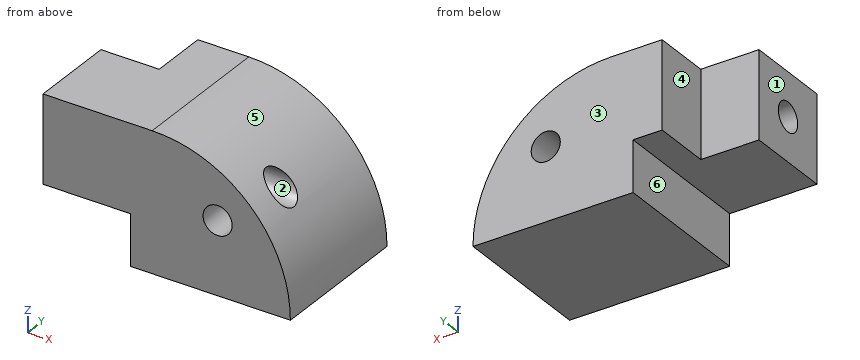
from build123d import *

# Parameters (mm, degrees)
F0_W     = 127
F0_H     = 120.65
F1_DEPTH = 215.9
F2_W     = 76.2
F2_H     = 44.45
F3_DEPTH = 127
F4_W     = 50.8
F4_H     = 76.2
F5_DEPTH = 50.8
F8_D     = 25.4
F8_DEPTH = 127
F8_TIP   = 7.6309298617
F9_R     = 120.64999
F10_D    = 25.4


# Not quite as in the source:
# - a fillet or chamfer is up to 0.001 mm smaller than in the source, because OpenCascade refuses the exact size


with BuildPart() as f1:
    # F0 (on Right) → F1 (new body)
    with BuildSketch(Plane.YZ):
        Rectangle(F0_W, F0_H)
    extrude(amount=F1_DEPTH)

    # F2 (on face) → F3 (cut)
    with BuildSketch(Plane.XZ.offset(63.5)):
        with Locations((38.1, -38.1)):
            Rectangle(F2_W, F2_H)
    extrude(amount=-F3_DEPTH, mode=Mode.SUBTRACT)

    # F4 (on face) → F5 (cut)
    with BuildSketch(Plane(origin=(0, 0, 0), x_dir=(0, -1, 0), z_dir=(-1, 0, 0))):
        with Locations((-38.1, 22.225)):
            Rectangle(F4_W, F4_H)
    extrude(amount=-F5_DEPTH, mode=Mode.SUBTRACT)

    # F8
    with Locations(Plane.XZ.offset(63.5)):
        with Locations((152.4, 3.175)):
            Hole(F8_D / 2, depth=F8_DEPTH)
            with Locations((0, 0, -(F8_DEPTH + F8_TIP / 2))):  # 118° drill point
                Cone(0, F8_D / 2, F8_TIP, mode=Mode.SUBTRACT)

    # F9 (radius 120.65 in the source; OpenCascade refuses exactly that, so slightly less here)
    f9_edges = [f1.edges().sort_by_distance(p)[0] for p in [
        (215.9, 0, 60.325),
    ]]
    fillet(f9_edges, radius=F9_R)

    # F10 (through all)
    with Locations(Plane(origin=(0, 0, 0), x_dir=(0, -1, 0), z_dir=(-1, 0, 0))):
        with Locations((25.4, 22.225)):
            Hole(F10_D / 2)


solid = f1.part
Could you check a few things on this model? Use its own coordinates, in mm. Face numbers are marked on the shaded views. A direction names the side the tool comes from. Give positions to 0.01 mm unless a question says otherwise; leave off trailing zeros. Loops run counter-clockwise (first coordinate to the right, second up) from the corner with the lowest first, then second, coordinate; pieces in that order, holes last. Notation, with made-up numbers: M -28,-35 L -1,-35 A11 ccw -1,-20 Z; hole C 63.25,49 d11. An arc over 180 degrees is marked long. Answer as a JSON object with one key per item and string values.
Q1. For the marked faces 4, 5 and 6, which set-ups out of +Z, -Z, +X, -X, +Y, -Y let a thin tool reach every point of the face, with its end or its side?
Values found:
{"face 4": "+Z, -Z, -X, +Y", "face 5": "+Z, +X, +Y, -Y", "face 6": "-Z, -X, +Y, -Y"}
Q2. If we mould it in two halves opening along Y, with no side actions, what happens to the marked faces 1, 2 and 3? For each: pulls with the +Y half, pulls with the -Y half, needs draft (parallel to the pull), parting line crosses it, or undercut.
Values found:
{"face 1": "needs draft", "face 2": "undercut", "face 3": "pulls with the +Y half"}
Q3. Suppose I cut it at D-D, the plane z = 44. List the corners of the cut face in (x, y) for me.
Values found:
{"outline": "M 0,-63.5 L 155.85,-63.5 L 155.85,63.5 L 50.8,63.5 L 50.8,12.7 L 0,12.7 Z"}
Q4. Suppose I cut it at C-C, the plane x = 152.4. List the corners of the cut face in (y, z) for me (3 decimals), plus the area to 3 significant figures.
Values found:
{"outline": "M -63.5,-60.325 L 63.5,-60.325 L 63.5,-9.525 L -63.5,-9.525 Z; M -63.5,15.875 L -36.399,15.875 A12.7 cw long -14.401,15.875 L 63.5,15.875 L 63.5,45.931 L -63.5,45.931 Z", "area": "9,860 mm²"}
Q5. For P1, Ø13.5, axis at y = 11, z = -33, coming from the -X side, with a flat end and sliding along its axis, tell me the tip position at first contact or that it passes through.
Values found:
{"P1": "stops at x = 76.2"}
Q6. If I drill on probe 1 along Z at (x, y) = (96, -25.4) (3 decimals); probe 2 along Z at (x, y) = (52, -25) (3 decimals); probe 3 along Z at (x, y) = (76, -2.5) (3 decimals), over which ranges is the centre line in solid material (lowest first)? Write a range as [from, to].
Values found:
{"probe 1": "z = [-60.325, 9.525], [34.925, 60.323]", "probe 2": "z = [-15.875, 9.531], [34.919, 60.325]", "probe 3": "z = [-15.875, 60.325]"}
